Geometry: see drawing. Coordinates: mm, zero at the bounding-box minimum. A direction names the side the tool comes from. Coordinates: 2 decimals unless noted, no trailing zeros. Write each loop counter-clockwise with the first axis right and the second up, starting at its lowest first coordinate (ties: lowest second). Pieces come first, ordered by that corner, then holes. Notation, with made-up numbers: M -24.75,47 L 14.25,47 A30 cw 14.25,69 Z; hole C 28,57 d9. An arc over 180 degrees is marked long. One line per item, written item: value. Start each with the question number.
Item 1: Cut plane B-B, the plane x = 27.5. Output: boundary loops of the cut face in (y, z), then the cut area to 3 significant figures.
Item 2: Set-up query: the marked faces 4 and 5. Return all of +Z, -Z, +X, -X, +Y, -Y with unobstructed straight access to the full face (end or side cutting, diameter ignored); none if empty.
Item 3: Mould query, pull axis Y, two halves, no side actions, for the marked faces 1, 2 and 3. Classes: released by +Y, released by -Y, zero draft, split by the parting line, or undercut.
Item 4: Cut plane A-A, the plane y = 23.75. Output: boundary loops of the cut face in (x, z).
Item 5: Ray query, L1, parallel to Z at x = 7, y = 2.5; L2, parallel to Y at x = 34.5, z = 39 (1 decimal); L3, parallel to X at y = 13.25, z = 54. Return the intervals inside material, ascending. Write a range as from..to.
Item 6: Pin query (flat end, axial travel): P1, Ø6, axis at x = 37, z = 53, coming from the +Y side; P2, Ø1, axis at y = 10, z = 55, coming from the -X side; P3, Ø3.5, axis at x = 47.5, y = 14, coming from the +Z side. Return the tip coordinate at first contact, or that it passes through.
Item 7: Cut plane C-C, the plane z = 50.5. Output: boundary loops of the cut face in (x, y).
Item 8: Cut plane D-D, the plane y = 15. Output: boundary loops of the cut face in (x, z).
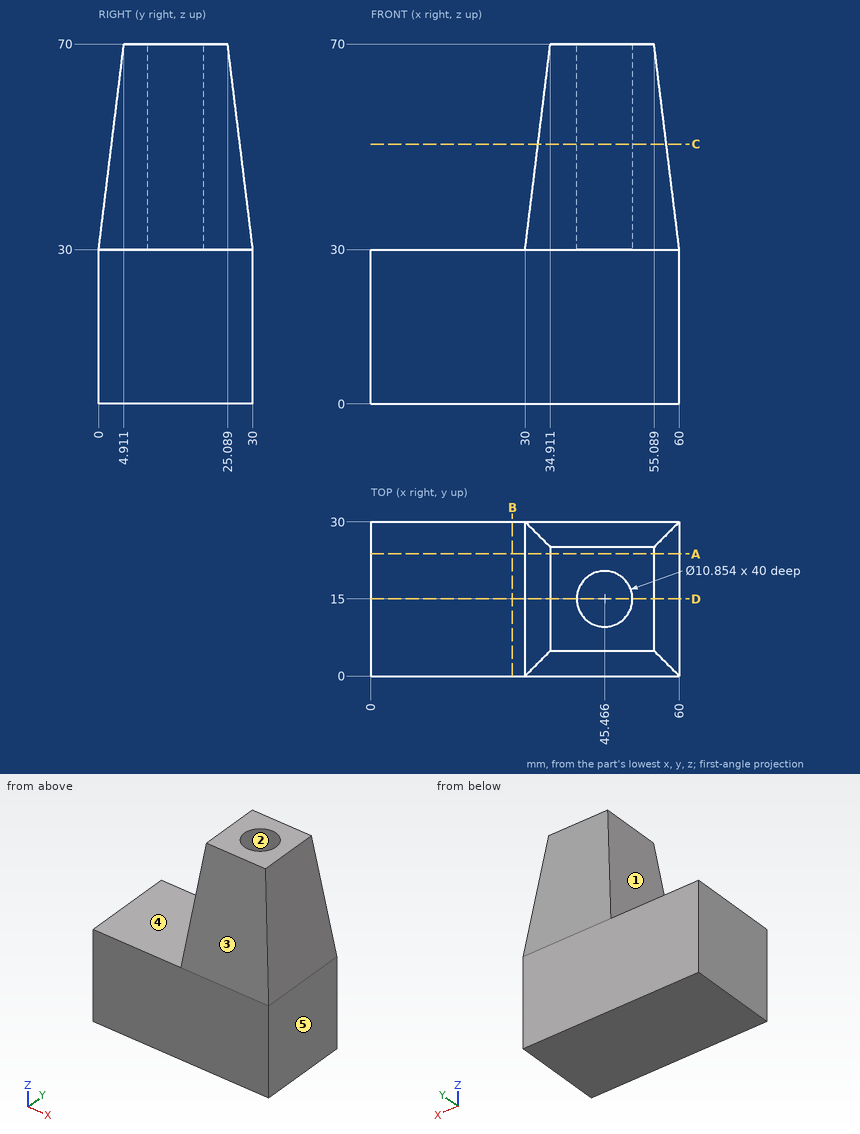
From the geometry:
1. outline: M 0,0 L 30,0 L 30,30 L 0,30 Z
1. area: 900 mm²
2. face 4: +Z, -X, +Y, -Y
2. face 5: +Z, -Z, +X, +Y, -Y
3. face 1: zero draft
3. face 2: undercut
3. face 3: released by -Y
4. outline: M 0,0 L 60,0 L 60,30 L 55.09,70 L 34.91,70 L 30,30 L 0,30 Z
5. L1: z = 0..30
5. L2: y = 1.1..28.9
5. L3: x = 32.95..40.33, 50.6..57.05
6. P1: stops at y = 27.54
6. P2: stops at x = 33.01
6. P3: stops at z = 30
7. outline: M 32.52,2.52 L 57.48,2.52 L 57.48,27.48 L 32.52,27.48 Z; hole C 45.47,15 d10.85
8. outline: M 0,0 L 60,0 L 60,30 L 55.09,70 L 50.89,70 L 50.89,30 L 40.04,30 L 40.04,70 L 34.91,70 L 30,30 L 0,30 Z
